Here's how the part is built. I have some questions about the finished solid (model axes, mm). A direction names the side the tool comes from. Give positions to 0.01 mm unless a question says otherwise; leave off trailing zeros. Loops run counter-clockwise (first coordinate to the right, second up) from the corner with the lowest first, then second, coordinate; pieces in that order, holes last. Notation, with made-up numbers: (5.25, -21.75) - (14.25, -21.75) arc R27 cw to (14.25, 4.25) - close; hole circle Ø9 at (12.5, 47). An arc over 180 degrees is marked (long way). Return JSON: item names as keys, results as strings. Group by question number.
(1) If we section it at A-A (z = 0): Please give me the cut outline in (x, y), then the cut area to 3 significant figures.
(2) If we section it at C-C (x = 2.3): Please give me the cut outline in (y, z), then the cut area to 3 significant figures.
(3) For P1, Ø3, axis at y = -1, z = 0, coming from the -X side; P2, Ø1.5, axis at y = 0, z = 9.57, coming from the +X side; P3, Ø3, axis at y = 0, z = 5, coming from the -X side, each with a flat end and sliding along its axis, tell me the tip position at first contact or that it passes through.
(4) If we section it at D-D (y = 0): State how many separate pieces and enclosed holes the cut face has, then the cut area to 3 significant figures.
(5) If we mould it in two halves opening along Z, with no side actions, what happens to faces 4 (the flat face through (1.6, -1, 9)), 5 (the cylindrical face through (0.79, 0.19, 8.96)), 6 (the cylindrical face through (0.8, 0, 17.5))? For each: released by +Z, released by -Z, zero draft, split by the parting line, or undercut.
(6) On a 3-axis mill with a long thin cutter (end or side, diameter ignored), from which of +Z, -Z, +X, -X, +Y, -Y can I reach the whole of each face in a straight line? I mean faces 1 (the cylindrical face through (0.79, 1.09, 0.14)), 2 (the flat face through (0, -1, -1)), 3 (the flat face through (1.6, -1, -1)). Say none if no direction works.
(7) I need wall thicknesses on probe 1 along X at (y, z) = (1.5, 6.25); probe 2 along Z at (x, y) = (0.25, -0.4); probe 3 along Y at (x, z) = (2.5, 0.75). Which ranges of each line are inside material? Lowest first, please. Write a range as [from, to].
(8) If we section it at B-B (y = 2.3): Please give me the cut outline in (x, z), then the cut area to 3 significant figures.
```python
from build123d import *

# Parameters (mm, degrees)
SKETCH1_R           = 1.1
SKETCH1_R_2         = 0.635
BOSS_EXTRUDE1_DEPTH = 1.6
SKETCH2_R           = 3
SKETCH2_R_2         = 2
BOSS_EXTRUDE2_DEPTH = 1.016
BOSS_EXTRUDE3_START = 0.762
SKETCH3_R           = 3
SKETCH3_R_2         = 2
BOSS_EXTRUDE3_DEPTH = 0.762


with BuildPart() as part:
    # Sketch1 → Boss-Extrude1 (new body)
    with BuildSketch(Plane.YZ):
        with BuildLine():
            Line((-2.98678731, 0.28125), (-1.493393655, 16.140625))
            ThreePointArc((-1.493393655, 16.140625), (0, 17.5), (1.493393655, 16.140625))
            Line((1.493393655, 16.140625), (2.98678731, 0.28125))
            ThreePointArc((2.98678731, 0.28125), (0, -3), (-2.98678731, 0.28125))
        make_face()
        with Locations(Location((0, 0, 0), (0, 0, 270))):
            Circle(SKETCH1_R, mode=Mode.SUBTRACT)
        with Locations(Location((0, 16, 0), (0, 0, 270))):
            Circle(SKETCH1_R_2, mode=Mode.SUBTRACT)
        with Locations(Location((0, 12.783333333, 0), (0, 0, 270))):
            Circle(SKETCH1_R_2, mode=Mode.SUBTRACT)
        with Locations(Location((0, 9.566666667, 0), (0, 0, 270))):
            Circle(SKETCH1_R_2, mode=Mode.SUBTRACT)
        with Locations(Location((0, 6.35, 0), (0, 0, 270))):
            Circle(SKETCH1_R_2, mode=Mode.SUBTRACT)
    extrude(amount=BOSS_EXTRUDE1_DEPTH)

    # Sketch2 → Boss-Extrude2 (add)
    with BuildSketch(Plane.YZ.offset(1.6)):
        with Locations(Location((0, 0, 0), (0, 0, 5.379378991))):
            Circle(SKETCH2_R)
        with Locations(Location((0, 0, 0), (0, 0, 270))):
            Circle(SKETCH2_R_2, mode=Mode.SUBTRACT)
    extrude(amount=BOSS_EXTRUDE2_DEPTH)

    # Sketch3 → Boss-Extrude3 (add)
    with BuildSketch(Plane(origin=(0, 0, 0), x_dir=(0, -1, 0), z_dir=(-1, 0, 0)).offset(BOSS_EXTRUDE3_START)):
        with Locations(Location((0, 0, 0), (0, 0, 90))):
            Circle(SKETCH3_R)
        with Locations(Location((0, 0, 0), (0, 0, 270))):
            Circle(SKETCH3_R_2, mode=Mode.SUBTRACT)
    extrude(amount=-BOSS_EXTRUDE3_DEPTH)


solid = part.part
```
Values:
{
 "1": {"outline": "(-0.76, -3) - (2.62, -3) - (2.62, -2) - (1.6, -2) - (1.6, -1.1) - (0, -1.1) - (0, -2) - (-0.76, -2) - close; (-0.76, 2) - (0, 2) - (0, 1.1) - (1.6, 1.1) - (1.6, 2) - (2.62, 2) - (2.62, 3) - (-0.76, 3) - close", "area": "9.64 mm2"},
 "2": {"outline": "circle Ø6 at (0, 0); hole circle Ø4 at (0, 0)", "area": "15.7 mm2"},
 "3": {"P1": "x = -0.76", "P2": "x = 1.6", "P3": "x = 0"},
 "4": {"separate pieces": "6", "enclosed holes": "0", "area": "24.7 mm2"},
 "5": {"face 4": "zero draft", "face 5": "undercut", "face 6": "released by +Z"},
 "6": {"face 1": "+X, -X", "face 2": "-X", "face 3": "+X"},
 "7": {"probe 1": "[0, 1.6]", "probe 2": "[-2.97, -1.02], [1.02, 5.86], [6.84, 9.07], [10.06, 12.29], [13.28, 15.51], [16.49, 17.45]", "probe 3": "[-2.9, -1.85], [1.85, 2.9]"},
 "8": {"outline": "(-0.76, -1.93) - (2.62, -1.93) - (2.62, 1.93) - (1.6, 1.93) - (1.6, 7.57) - (0, 7.57) - (0, 1.93) - (-0.76, 1.93) - close", "area": "22.1 mm2"}
}
